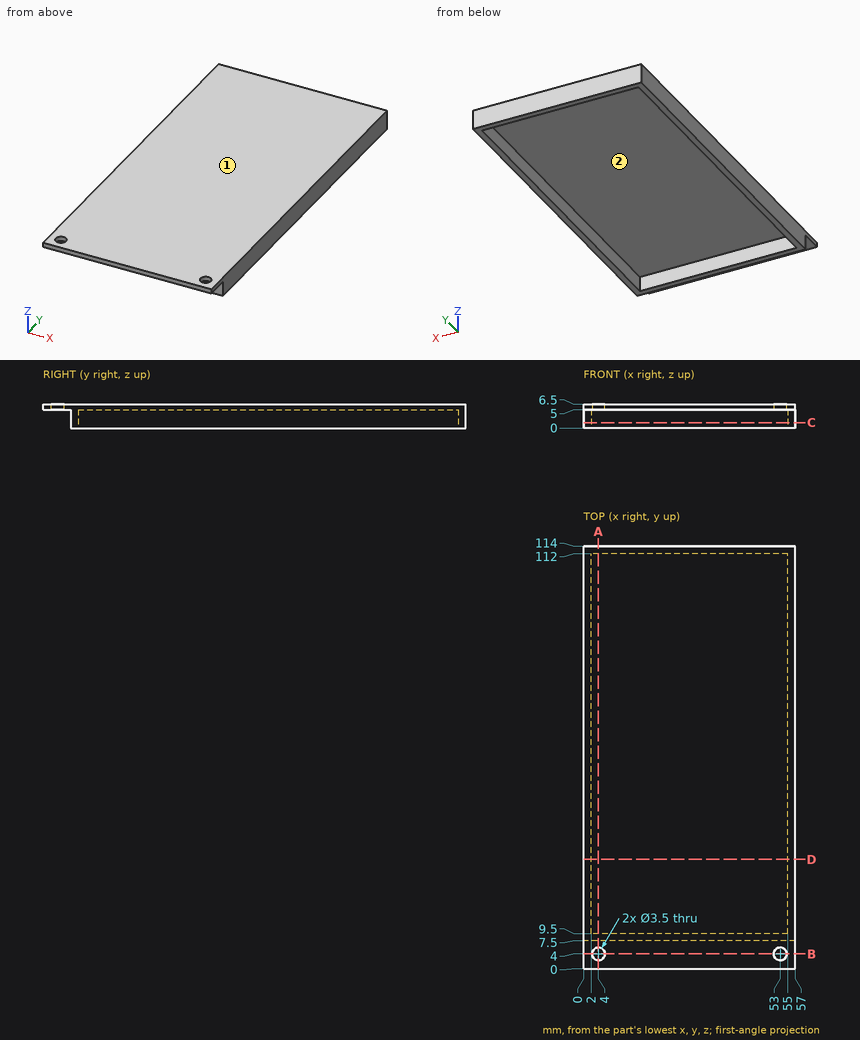
Part print with two shaded views. Sizes in mm from the minimum x, y, z corner. Round coordinates to 2 decimals unless told otherwise and drop trailing zeros. Write each loop counter-clockwise with the first axis right and the second up, starting at its lowest first coordinate (ties: lowest second). Pieces come first, ordered by that corner, then holes. Notation, with made-up numbers: M 15,12 L 39,12 A17 ccw 39,34 Z; hole C 57.5,88.5 d8. An arc over 180 degrees is marked long. Put each result on its own line as item: value. Start each with the question number.
1) Saw through at B-B, the plane y = 4. Write the cut outline in (x, z), and give its area (3 significant figures).
2) Drill centre lines: probe 1 along Y at (x, z) = (22.5, 3.25); probe 2 along Y at (x, z) = (53, 5.6); probe 3 along X at (y, z) = (46.5, 1). Where is each one in solid material? Low to high. Write a range as [from, to].
3) Pin check, flat tips, straight feed: pin 1 Ø2.5 at (x, z) = (38.5, 1.5) entering from -Y; pin 2 Ø3 at (x, y) = (53, 4) entering from +Z; pin 3 Ø16 at (x, y) = (37, 43) entering from -Z. Stop position of each tip, or through.
4) Saw through at A-A, the plane x = 4. Write the cut outline in (y, z).
5) Saw through at C-C, the plane z = 1.5. Write the cut outline in (x, y), and give its area (3 significant figures).
6) Saw through at D-D, the plane y = 29.5. Write the cut outline in (x, z).
7) Pull direction X, two halves, no side cores. Call the marked faces 1 and 2: pulls with the +X half, pulls with the -X half, needs draft (parallel to the pull), parting line crosses it, or undercut.
Resolved:
1. outline: M 0,5 L 2.25,5 L 2.25,6.5 L 0,6.5 Z; M 5.75,5 L 51.25,5 L 51.25,6.5 L 5.75,6.5 Z; M 54.75,5 L 57,5 L 57,6.5 L 54.75,6.5 Z
1. area: 75.0 mm²
2. probe 1: [7.5, 9.5], [112, 114]
2. probe 2: [0, 2.25], [5.75, 114]
2. probe 3: [0, 2], [55, 57]
3. pin 1: y = 7.5
3. pin 2: through
3. pin 3: z = 5
4. outline: M 0,5 L 2.25,5 L 2.25,6.5 L 0,6.5 Z; M 5.75,5 L 7.5,5 L 7.5,0 L 9.5,0 L 9.5,5 L 112,5 L 112,0 L 114,0 L 114,6.5 L 5.75,6.5 Z
5. outline: M 0,7.5 L 57,7.5 L 57,114 L 0,114 Z; hole M 2,9.5 L 55,9.5 L 55,112 L 2,112 Z
5. area: 638 mm²
6. outline: M 0,0 L 2,0 L 2,5 L 55,5 L 55,0 L 57,0 L 57,6.5 L 0,6.5 Z
7. face 1: needs draft
7. face 2: undercut
